The model under review builds one solid part; all positions refer to its coordinate system, in mm. Face numbers are marked on the shaded views. A direction names the side the tool comes from. Round coordinates to 2 decimals unless told otherwise and drop trailing zeros. Loops run counter-clockwise (first coordinate to the right, second up) from the corner with the lowest first, then second, coordinate; pieces in that order, holes last. Notation, with made-up numbers: M 13,-34.75 L 54,-34.75 A18 cw 54,-12.75 Z; hole C 16,-3 d7. An arc over 180 degrees is marked long. Return JSON: item names as keys, results as strings. Group by question number.
Q1. Consider section A-A (x = -85). State the section outline as (y, z) points, and give its area (4 significant figures).
Q2. Consider section C-C (y = 13.5). State the section outline as (x, z) points, and give its area (3 significant figures).
Q3. Clearance check with flat-ended pins moving along their axes: pin 1 Ø1.5 at (y, z) = (69, 27.5) entering from -X; pin 2 Ø1 at (x, z) = (-1.5, 25.5) entering from -Y; pin 3 Ø5 at (x, z) = (-89, -0.5) entering from -Y; pin 4 Ø16 at (x, y) = (-90.5, 61.5) entering from +Z. State where each tip first meets the part, or that it passes through.
Q4. To check wall thickness, follow line 1 along X through (y, z) = (103.85, 34.65); line 2 along Z through (x, y) = (63, 32.5). State the ranges of each line that lie inside material, in increasing order.
Q5. Draft analysis for pull direction X (two halves, no side actions). For the marked faces 3, 4, 5 and 6, state which applies: pulls with the +X half, pulls with the -X half, needs draft (parallel to the pull), parting line crosses it, or undercut.
Q6. Consider section B-B (z = -14.85). State the section outline as (x, y) points, and give its area (3 significant figures).
Q7. Consider section D-D (x = 2). State the section outline as (y, z) points.
Q8. For the marked faces 1 and 2, list the 3-axis set-ups (+Z, -Z, +X, -X, +Y, -Y) from which the entire face can be reached by the end or side of a thin tool; tool diameter is ignored.
from build123d import *

# Parameters (mm, degrees)
SKETCH1_W           = 150
SKETCH1_H           = 150
BOSS_EXTRUDE1_DEPTH = 10
BOSS_EXTRUDE2_DEPTH = 100
BOSS_EXTRUDE3_DEPTH = 30
SKETCH9_R           = 2.55
SKETCH9_W           = 20
SKETCH9_H           = 40
CUT_EXTRUDE1_DEPTH  = 5
BOSS_EXTRUDE4_DEPTH = 25
SKETCH12_W          = 110
SKETCH12_H          = 5
BOSS_EXTRUDE5_DEPTH = 8
FILLET2_R           = 50
CUT_EXTRUDE3_DEPTH  = 8
BOSS_EXTRUDE6_DEPTH = 18
SKETCH15_W          = 150
SKETCH15_H          = 150
BOSS_EXTRUDE7_DEPTH = 5
SKETCH16_W          = 150
SKETCH16_H          = 23
CUT_EXTRUDE4_DEPTH  = 75


with BuildPart() as part:
    # Sketch1 → Boss-Extrude1 (new body)
    with BuildSketch(Plane(origin=(0, 0, 0), x_dir=(1, 0, 0), z_dir=(0, 1, 0))):
        Rectangle(SKETCH1_W, SKETCH1_H)
    extrude(amount=BOSS_EXTRUDE1_DEPTH)

    # Sketch2 → Boss-Extrude2 (add)
    with BuildSketch(Plane(origin=(0, 10, 0), x_dir=(1, 0, 0), z_dir=(0, 1, 0))):
        Polygon((-75, 75), (75, 75), (75, -75), (60, -75), (60, -70), (70, -70), (70, 70), (-70, 70), (-70, -70), (-60, -70), (-60, -75), (-75, -75), align=None)
    extrude(amount=BOSS_EXTRUDE2_DEPTH)

    # Sketch8 → Boss-Extrude3 (add)
    with BuildSketch(Plane.ZY.offset(75)):
        Polygon((9.9, 106), (39.9, 106), (39.9, 101), (-20.1, 101), (-20.1, 106), align=None)
    extrude(amount=BOSS_EXTRUDE3_DEPTH)

    # Sketch9 → Cut-Extrude1 (cut)
    with BuildSketch(Plane(origin=(0, 106, 0), x_dir=(1, 0, 0), z_dir=(0, 1, 0))):
        with Locations(Location((-95, 14.85, 0), (0, 0, 270))):
            Circle(SKETCH9_R)
        with Locations(Location((-85, 14.85, 0), (0, 0, 90))):
            Circle(SKETCH9_R)
        with Locations(Location((-85, -34.65, 0), (0, 0, 270))):
            Circle(SKETCH9_R)
        with Locations(Location((-95, -34.65, 0), (0, 0, 90))):
            Circle(SKETCH9_R)
        with Locations((-90, -9.9)):
            Rectangle(SKETCH9_W, SKETCH9_H)
    extrude(amount=-CUT_EXTRUDE1_DEPTH, mode=Mode.SUBTRACT)

    # Sketch10 → Boss-Extrude4 (add)
    with BuildSketch(Plane.ZY.offset(75)):
        Polygon((-10.1, 77.3), (-10.1, 72.3), (7.4, 72.3), (7.4, 52.3), (12.4, 52.3), (12.4, 72.3), (29.9, 72.3), (29.9, 77.3), align=None)
    extrude(amount=BOSS_EXTRUDE4_DEPTH)

    # Sketch12 → Boss-Extrude5 (add)
    with BuildSketch(Plane(origin=(-70, 0, 0), x_dir=(0, 0, -1), z_dir=(1, 0, 0))):
        with Locations((15, 100)):
            Rectangle(SKETCH12_W, SKETCH12_H)
    boss_extrude5 = extrude(amount=BOSS_EXTRUDE5_DEPTH)

    # Mirror1: Boss-Extrude5 across plane
    add(boss_extrude5.mirror(Plane(origin=(0, 0, 0), x_dir=(0, 0, 1), z_dir=(1, 0, 0))))

    # Fillet2
    # the kernel refuses this fillet: 50 mm, written as the material it takes off along each edge
    with BuildSketch(Plane(origin=(70, 102.5, 40), x_dir=(0, -1, 0), z_dir=(-1, 0, 0))) as fillet2_piece_1:
        with BuildLine():
            CenterArc((50, -21.794494718), FILLET2_R, 154.158067237, 25.841932763)
            Line((0, -21.794494718), (0, 0))
            Line((0, 0), (5, 0))
        make_face()
    extrude(amount=62.486236794, mode=Mode.SUBTRACT)
    with BuildSketch(Plane(origin=(-70, 102.5, 40), x_dir=(0, 0, -1), z_dir=(1, 0, 0))) as fillet2_piece_2:
        with BuildLine():
            CenterArc((21.794494718, -50), FILLET2_R, 90, 25.841932763)
            Line((0, -5), (0, 0))
            Line((0, 0), (21.794494718, 0))
        make_face()
    extrude(amount=62.486236794, mode=Mode.SUBTRACT)

    # Sketch13 → Cut-Extrude3 (cut)
    with BuildSketch(Plane.XY.offset(12.4)):
        Polygon((-100, 52.3), (-100, 70.3), (-80, 52.3), align=None)
    extrude(amount=-CUT_EXTRUDE3_DEPTH, mode=Mode.SUBTRACT)

    # Sketch14 → Boss-Extrude6 (add)
    with BuildSketch(Plane(origin=(0, 110, 0), x_dir=(1, 0, 0), z_dir=(0, 1, 0))):
        Polygon((-75, -75), (-60, -75), (-60, -70), (-70, -70), (-70, -35), (-75, -35), align=None)
        Polygon((60, -75), (60, -70), (70, -70), (70, 70), (-70, 70), (-70, 65), (-75, 65), (-75, 75), (75, 75), (75, -75), align=None)
    extrude(amount=BOSS_EXTRUDE6_DEPTH)

    # Sketch15 → Boss-Extrude7 (add)
    with BuildSketch(Plane(origin=(0, 128, 0), x_dir=(1, 0, 0), z_dir=(0, 1, 0))):
        Rectangle(SKETCH15_W, SKETCH15_H)
    extrude(amount=BOSS_EXTRUDE7_DEPTH)

    # Sketch16 → Cut-Extrude4 (cut, symmetric)
    with BuildSketch(Plane.XY):
        with Locations((0, 121.5)):
            Rectangle(SKETCH16_W, SKETCH16_H)
    extrude(amount=CUT_EXTRUDE4_DEPTH, both=True, mode=Mode.SUBTRACT)


solid = part.part
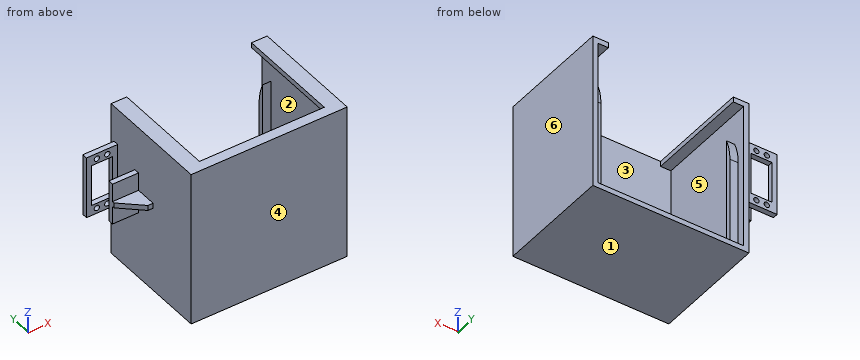
Values:
{
 "1": {"outline": "M 56.8,7.4 L 72.3,7.4 L 72.3,-10.1 L 77.3,-10.1 L 77.3,29.9 L 72.3,29.9 L 72.3,12.4 L 56.8,12.4 Z; M 101,-20.1 L 106,-20.1 L 106,-17.4 L 101,-17.4 Z; M 101,-12.3 L 106,-12.3 L 106,-10.1 L 101,-10.1 Z; M 101,29.9 L 106,29.9 L 106,32.1 L 101,32.1 Z; M 101,37.2 L 106,37.2 L 106,39.9 L 101,39.9 Z", "area": "326.5 mm2"},
 "2": {"outline": "M -75,-75 L 75,-75 L 75,75 L 60,75 L 60,70 L 70,70 L 70,-70 L -70,-70 L -70,70 L -60,70 L -60,75 L -75,75 Z", "area": "2,300 mm2"},
 "3": {"pin 1": "stops at x = -75", "pin 2": "stops at y = 0", "pin 3": "stops at y = 72.3", "pin 4": "stops at z = 12.4"},
 "4": {"line 1": "x = -105 to -97.55, -92.45 to -87.55, -82.45 to -70, 70 to 75", "line 2": "z = -75 to -70, 70 to 75"},
 "5": {"face 3": "undercut", "face 4": "needs draft", "face 5": "undercut", "face 6": "pulls with the +X half"},
 "6": {"outline": "M -105,101 L -97.55,101 L -97.55,106 L -105,106 Z; M -92.45,101 L -87.55,101 L -87.55,106 L -92.45,106 Z; M -82.45,101 L -75,101 L -75,0 L 75,0 L 75,110 L 70,110 L 70,102.5 L 62,102.5 L 62,97.5 L 70,97.5 L 70,10 L -70,10 L -70,97.5 L -62,97.5 L -62,102.5 L -70,102.5 L -70,110 L -75,110 L -75,106 L -82.45,106 Z", "area": "2,680 mm2"},
 "7": {"outline": "M 0,-75 L 110,-75 L 110,-70 L 10,-70 L 10,75 L 0,75 Z"},
 "8": {"face 1": "-Z, +X, -X, +Y, -Y", "face 2": "none"}
}
